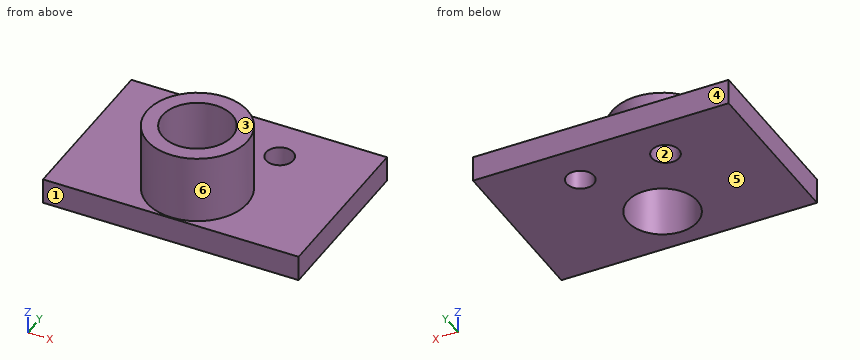
from build123d import *

# Parameters (mm, degrees)
SKETCH_1_W      = 30
SKETCH_1_H      = 20
SKETCH_1_R      = 1.6
SKETCH_1_R_2    = 4.1
EXTRUDE_1_DEPTH = 3
SKETCH_2_R      = 5.9
SKETCH_2_R_2    = 4.1
EXTRUDE_2_DEPTH = 8


with BuildPart() as part:
    # 草图1 → 凸台-拉伸1 (new body)
    with BuildSketch(Plane.XY):
        with Locations((-3.612174849, 26.048923765)):
            Rectangle(SKETCH_1_W, SKETCH_1_H)
        with Locations((-8.612174849, 31.048923765)):
            Circle(SKETCH_1_R, mode=Mode.SUBTRACT)
        with Locations((1.387825151, 31.048923765)):
            Circle(SKETCH_1_R, mode=Mode.SUBTRACT)
        with Locations((-3.612174849, 22.073206433)):
            Circle(SKETCH_1_R_2, mode=Mode.SUBTRACT)
    extrude(amount=EXTRUDE_1_DEPTH)

    # 草图2 → 凸台-拉伸2 (add)
    with BuildSketch(Plane.XY.offset(3)):
        with Locations((-3.612174849, 22.073206433)):
            Circle(SKETCH_2_R)
        with Locations((-3.612174849, 22.073206433)):
            Circle(SKETCH_2_R_2, mode=Mode.SUBTRACT)
    extrude(amount=EXTRUDE_2_DEPTH)


solid = part.part
Verification items for the finished model (mm, model axes). Face numbers are marked on the shaded views. A direction names the side the tool comes from. Give positions to 0.01 mm unless a question says otherwise; leave off trailing zeros. Loops run counter-clockwise (first coordinate to the right, second up) from the corner with the lowest first, then second, coordinate; pieces in that order, holes last. Notation, with made-up numbers: (-6.75, -38) - (15.25, -38) arc R17 ccw to (15.25, -34) - close; hole circle Ø3 at (14, 74). An arc over 180 degrees is marked (long way). Write item = value, one per line. Start each with the question number.
Q1. Mould release check, pull along Y, two halves, no side actions. Record for the marked faces 1, 2, 3 and 4: released by +Y, released by -Y, zero draft, split by the parting line, or undercut.
Q2. Cross-section at B-B, the plane x = 1.75. Enter the section's corners in (y, z).
Q3. Cross-section at A-A, the plane y = 19.75. Enter the section's corners in (x, z), and give its area (3 significant figures).
Q4. Depth check by flat-ended pin: P1, Ø3.5, axis at x = 1.39, y = 31.05, coming from the +Z side; P2, Ø9.5, axis at x = -3.61, y = 22.07, coming from the +Z side; P3, Ø1, axis at y = 27, z = 5.5, coming from the -X side. Enter the tip coordinate at first touch or a pass-through.
Q5. Cross-section at C-C, the plane z = 2.5. Enter the section's corners in (x, y).
Q6. Cross-section at D-D, the plane y = 33.25. Enter the section's corners in (x, z).
Q7. Thickness scan on line 1 (Y direction, x = -3.75, z = 6.5); line 2 (Z direction, x = -10, y = 26.75); line 3 (Y direction, x = -4.75, z = 1). Record the ranges inside material, lowest first.
Q8. Tool access check on the marked faces 5 and 6. Record the directions out of +Z, -Z, +X, -X, +Y, -Y that give a thin tool (end or side, any length) a straight path to the whole face; none if there is none.
Answer key:
q1.face_1 = released by -Y
q1.face_2 = undercut
q1.face_3 = zero draft
q1.face_4 = released by +Y
q2.outline = (16.05, 0) - (29.49, 0) - (29.49, 3) - (24.53, 3) - (24.53, 11) - (19.61, 11) - (19.61, 3) - (16.05, 3) - close; (32.61, 0) - (36.05, 0) - (36.05, 3) - (32.61, 3) - close
q3.outline = (-18.61, 0) - (-6.99, 0) - (-6.99, 11) - (-9.04, 11) - (-9.04, 3) - (-18.61, 3) - close; (-0.23, 0) - (11.39, 0) - (11.39, 3) - (1.81, 3) - (1.81, 11) - (-0.23, 11) - close
q3.area = 102 mm^2
q4.P1 = 3
q4.P2 = 11
q4.P3 = -7.51
q5.outline = (-18.61, 16.05) - (11.39, 16.05) - (11.39, 36.05) - (-18.61, 36.05) - close; hole circle Ø3.2 at (-8.61, 31.05); hole circle Ø8.2 at (-3.61, 22.07); hole circle Ø3.2 at (1.39, 31.05)
q6.outline = (-18.61, 0) - (11.39, 0) - (11.39, 3) - (-18.61, 3) - close
q7.line_1 = 16.17 to 17.98, 26.17 to 27.97
q7.line_2 = 0 to 3
q7.line_3 = 16.05 to 18.13, 26.01 to 36.05
q8.face_5 = -Z, +X, -X, +Y, -Y
q8.face_6 = +Z
